from build123d import *

# Parameters (mm, degrees)
F0_W     = 24.4
F0_H     = 24.4
F0_W_2   = 18.4
F0_H_2   = 18.4
F1_DEPTH = 3
F2_W     = 24.4
F2_H     = 24.4
F2_W_2   = 12.4
F2_H_2   = 12.4
F3_DEPTH = 3
F4_W     = 24.4
F4_H     = 3
F5_DEPTH = 5


with BuildPart() as f1:
    # F0 (on Top) → F1 (new body)
    with BuildSketch(Plane.XY):
        Rectangle(F0_W, F0_H)
        Rectangle(F0_W_2, F0_H_2, mode=Mode.SUBTRACT)
    extrude(amount=F1_DEPTH)

    # F2 (on face) → F3 (join)
    with BuildSketch(Plane(origin=(0, 0, 0), x_dir=(1, 0, 0), z_dir=(0, 0, -1))):
        Rectangle(F2_W, F2_H)
        Rectangle(F2_W_2, F2_H_2, mode=Mode.SUBTRACT)
    extrude(amount=F3_DEPTH)

    # F4 (on face) → F5 (join)
    with BuildSketch(Plane.XY.offset(3)):
        with Locations((0, -10.7)):
            Rectangle(F4_W, F4_H)
        with Locations((0, 10.7)):
            Rectangle(F4_W, F4_H)
    extrude(amount=F5_DEPTH)


solid = f1.part
Geometry check sheet. Reference: the model listing, model coordinates, mm. A direction names the side the tool comes from. Give positions to 0.01 mm unless a question says otherwise; leave off trailing zeros. Loops run counter-clockwise (first coordinate to the right, second up) from the corner with the lowest first, then second, coordinate; pieces in that order, holes last. Notation, with made-up numbers: M 48.5,42 L 56.5,42 A17 ccw 56.5,56 Z; hole C 44.25,62.25 d6. An arc over 180 degrees is marked long. Write each question's results on one line, items separated by ' | '.
1) Tool access check on faces 1 (the face through (-9.2, 0, 1)), 2 (the face through (0, -6.2, -1)), 3 (the face through (-11, 0, 3)). Record the directions out of +Z, -Z, +X, -X, +Y, -Y that give a thin tool (end or side, any length) a straight path to the whole face; none if there is none.
Answers follow:
face 1: +Z | face 2: +Z, -Z | face 3: +Z, +X, -X
2) Thickness scan on line 1 (Y direction, x = -9, z = 5.25); line 2 (Y direction, x = -2.25, z = -1). Record the ranges inside material, lowest first.
Answers follow:
line 1: -12.2 to -9.2, 9.2 to 12.2 | line 2: -12.2 to -6.2, 6.2 to 12.2
3) Section check D-D, the plane x = 4.5. Record the boundary of the cut face in (y, z), plus the area to 3 significant figures.
Answers follow:
outline: M -12.2,-3 L -6.2,-3 L -6.2,0 L -9.2,0 L -9.2,8 L -12.2,8 Z; M 6.2,-3 L 12.2,-3 L 12.2,8 L 9.2,8 L 9.2,0 L 6.2,0 Z | area: 84.0 mm2
4) Release check for a two-part mould opening along X. For faces 4 (the face through (-12.2, 0, 1)), 5 (the face through (6.2, 0, -1)), 6 (the face through (11, 0, 3)) record: +X half, -X half, draft (parallel to the pull), parting line (faces both ways), or undercut.
Answers follow:
face 4: -X half | face 5: undercut | face 6: draft
5) Section check A-A, the plane z = 7. Record the boundary of the cut face in (x, y), plus the area to 3 significant figures.
Answers follow:
outline: M -12.2,-12.2 L 12.2,-12.2 L 12.2,-9.2 L -12.2,-9.2 Z; M -12.2,9.2 L 12.2,9.2 L 12.2,12.2 L -12.2,12.2 Z | area: 146 mm2
6) Section check C-C, the plane z = 1.5. Record the boundary of the cut face in (x, y).
Answers follow:
outline: M -12.2,-12.2 L 12.2,-12.2 L 12.2,12.2 L -12.2,12.2 Z; hole M -9.2,-9.2 L 9.2,-9.2 L 9.2,9.2 L -9.2,9.2 Z
7) Gauge pin test, flat ends, axial feed: pin 1 (8 mm diameter, centred on x = -1, y = -7.5, fed in from +Z); pin 2 (0.9 mm diameter, centred on x = 10, y = 0, fed in from +Z); pin 3 (2 mm diameter, centred on x = -5, y = -3.5, fed in from -Z). Record the tip position at first contact, or that the pin passes through.
Answers follow:
pin 1: z = 8 | pin 2: z = 3 | pin 3: through
8) Section check B-B, the plane y = 4.75. Record the boundary of the cut face in (x, z).
Answers follow:
outline: M -12.2,-3 L -6.2,-3 L -6.2,0 L -9.2,0 L -9.2,3 L -12.2,3 Z; M 6.2,-3 L 12.2,-3 L 12.2,3 L 9.2,3 L 9.2,0 L 6.2,0 Z
